Can you work these out from the model? Positions are in its coordinate system, mm. Face numbers are marked on the shaded views. A direction names the side the tool comes from. Give positions to 0.01 mm unless a question says otherwise; leave off trailing zeros. Order: outer loops, then holes, each group sorted by start corner. A loop starts at its lowest first (then second) coordinate and runs counter-clockwise, first axis right, second up. Notation, with made-up numbers: (67.5, -7.5) - (103.5, -7.5) arc R26 cw to (103.5, 15.5) - close; hole circle Ø10 at (12.5, -15). An arc over 180 degrees is marked (long way). Write each question's results on one line, items separated by ' | '. Start each with the question number.
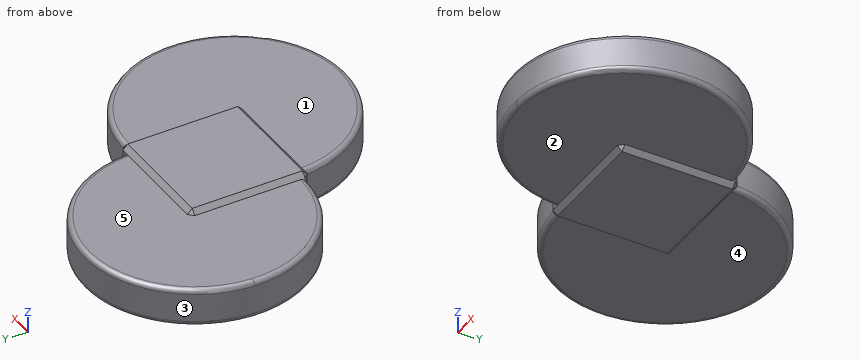
from build123d import *

# Parameters (mm, degrees)
F0_W          = 254
F0_H          = 254
F1_DEPTH      = 50.8
F1_DEPTH_BACK = 50.8
F2_SIZE       = 10.16
F1_FACE_W     = 233.68
F1_FACE_H     = 81.28
F1_FACE1_W    = 233.68
F1_FACE1_H    = 81.28
F5_T4_ANGLE   = 280.0079997231
F5_T9_ANGLE   = 280.0079997231
F5_T14_ANGLE  = 280.0079997231
F5_T19_ANGLE  = 280.0079997231
F5_T24_ANGLE  = 280.0079997231
F5_T29_ANGLE  = 280.0079997231
F5_T34_ANGLE  = 280.0079997231
F5_T39_ANGLE  = 280.0079997231
F5_T44_ANGLE  = 280.0079997231
F5_T49_ANGLE  = 280.0079997231
F5_T54_ANGLE  = 280.0079997231
F5_T59_ANGLE  = 280.0079997231


# Not quite as in the source:
# - a fillet or chamfer that OpenCascade refuses, or shapes differently, is made with other operations: its cross-section is extruded or revolved along the edge and cut away or added


with BuildPart() as f1:
    # F0 (on Top) → F1 (new body, two sides)
    with BuildSketch(Plane.XY) as f1_sk:
        Rectangle(F0_W, F0_H)
    extrude(amount=F1_DEPTH)
    extrude(f1_sk.sketch, amount=-F1_DEPTH_BACK)

    # F2
    f2_edges = [f1.edges().sort_by_distance(p)[0] for p in [
        (0, -127, 50.8),
        (127, -127, 0),
        (127, 0, 50.8),
        (-127, -127, 0),
        (0, -127, -50.8),
        (127, 0, -50.8),
        (127, 127, 0),
        (-127, 0, 50.8),
        (-127, 0, -50.8),
        (-127, 127, 0),
        (0, 127, 50.8),
        (0, 127, -50.8),
    ]]
    chamfer(f2_edges, length=F2_SIZE)

    # F1_face (on face) → F3 (revolve)
    with BuildSketch(Plane.YZ.offset(127)):
        Rectangle(F1_FACE_W, F1_FACE_H)
    revolve(axis=Axis((127, -116.84, 0), (0, 0, -1)))

    # F1_face1 (on face) → F4 (revolve)
    with BuildSketch(Plane(origin=(-127, 0, 0), x_dir=(0, -1, 0), z_dir=(-1, 0, 0))):
        Rectangle(F1_FACE1_W, F1_FACE1_H)
    revolve(axis=Axis((-127, 116.84, 0), (0, 0, 1)))

    # F5: fillet of radius 10.16 on 4 edges, made by hand


with BuildPart() as f5_tool2:
    # F5_s3 → F5_t4 (revolve)
    with BuildSketch(Plane(origin=(112.850510213, 12.3590473355, 0), x_dir=(0, 0, 1), z_dir=(-0.9940564274, -0.1088660602, 0))):
        with BuildLine():
            ThreePointArc((30.48, 103.70845737), (37.6642048969, 100.7326622668), (40.64, 93.54845737))
            Line((40.64, 93.54845737), (40.64, 103.70845737))
            Line((40.64, 103.70845737), (30.48, 103.70845737))
        make_face()
    revolve(axis=Axis((127, -116.84, 40.64), (0, 0, -1)), revolution_arc=F5_T4_ANGLE)

    split(bisect_by=Plane(origin=(83.82, 0, 83.82), x_dir=(0, 1, 0), z_dir=(0.7071067812, 0, 0.7071067812)), keep=Keep.TOP)


with BuildPart() as f1_1:
    add(f1.part)

    # F5_t1: cut F5_tool2
    add(f5_tool2.part, mode=Mode.SUBTRACT)


with BuildPart() as f5_tool7:
    # F5_s8 → F5_t9 (revolve)
    with BuildSketch(Plane(origin=(112.850510213, 12.3590473355, 0), x_dir=(0, 0, 1), z_dir=(-0.9940564274, -0.1088660602, 0))):
        with BuildLine():
            ThreePointArc((30.48, 103.70845737), (37.6642048969, 100.7326622668), (40.64, 93.54845737))
            Line((40.64, 93.54845737), (40.64, 103.70845737))
            Line((40.64, 103.70845737), (30.48, 103.70845737))
        make_face()
    revolve(axis=Axis((127, -116.84, 40.64), (0, 0, -1)), revolution_arc=F5_T9_ANGLE)

    split(bisect_by=Plane(origin=(121.92, 121.92, 0), x_dir=(0, 0, 1), z_dir=(0.7071067812, 0.7071067812, 0)), keep=Keep.TOP)


with BuildPart() as f1_2:
    add(f1_1.part)

    # F5_t6: cut F5_tool7
    add(f5_tool7.part, mode=Mode.SUBTRACT)


with BuildPart() as f5_tool12:
    # F5_s13 → F5_t14 (revolve)
    with BuildSketch(Plane(origin=(112.850510213, 12.3590473355, 0), x_dir=(0, 0, 1), z_dir=(-0.9940564274, -0.1088660602, 0))):
        with BuildLine():
            ThreePointArc((30.48, 103.70845737), (37.6642048969, 100.7326622668), (40.64, 93.54845737))
            Line((40.64, 93.54845737), (40.64, 103.70845737))
            Line((40.64, 103.70845737), (30.48, 103.70845737))
        make_face()
    revolve(axis=Axis((127, -116.84, 40.64), (0, 0, -1)), revolution_arc=F5_T14_ANGLE)

    split(bisect_by=Plane.XZ.offset(127), keep=Keep.TOP)


with BuildPart() as f1_3:
    add(f1_2.part)

    # F5_t11: cut F5_tool12
    add(f5_tool12.part, mode=Mode.SUBTRACT)


with BuildPart() as f5_tool17:
    # F5_s18 → F5_t19 (revolve)
    with BuildSketch(Plane(origin=(112.850510213, 12.3590473355, 0), x_dir=(0, 0, 1), z_dir=(-0.9940564274, -0.1088660602, 0))):
        with BuildLine():
            ThreePointArc((-30.48, 103.70845737), (-37.6642048969, 100.7326622668), (-40.64, 93.54845737))
            Line((-40.64, 93.54845737), (-40.64, 103.70845737))
            Line((-40.64, 103.70845737), (-30.48, 103.70845737))
        make_face()
    revolve(axis=Axis((127, -116.84, -40.64), (0, 0, -1)), revolution_arc=F5_T19_ANGLE)

    split(bisect_by=Plane(origin=(83.82, 0, -83.82), x_dir=(0, 1, 0), z_dir=(0.7071067812, 0, -0.7071067812)), keep=Keep.TOP)


with BuildPart() as f1_4:
    add(f1_3.part)

    # F5_t16: cut F5_tool17
    add(f5_tool17.part, mode=Mode.SUBTRACT)


with BuildPart() as f5_tool22:
    # F5_s23 → F5_t24 (revolve)
    with BuildSketch(Plane(origin=(112.850510213, 12.3590473355, 0), x_dir=(0, 0, 1), z_dir=(-0.9940564274, -0.1088660602, 0))):
        with BuildLine():
            ThreePointArc((-30.48, 103.70845737), (-37.6642048969, 100.7326622668), (-40.64, 93.54845737))
            Line((-40.64, 93.54845737), (-40.64, 103.70845737))
            Line((-40.64, 103.70845737), (-30.48, 103.70845737))
        make_face()
    revolve(axis=Axis((127, -116.84, -40.64), (0, 0, -1)), revolution_arc=F5_T24_ANGLE)

    split(bisect_by=Plane(origin=(121.92, 121.92, 0), x_dir=(0, 0, 1), z_dir=(0.7071067812, 0.7071067812, 0)), keep=Keep.TOP)


with BuildPart() as f1_5:
    add(f1_4.part)

    # F5_t21: cut F5_tool22
    add(f5_tool22.part, mode=Mode.SUBTRACT)


with BuildPart() as f5_tool27:
    # F5_s28 → F5_t29 (revolve)
    with BuildSketch(Plane(origin=(112.850510213, 12.3590473355, 0), x_dir=(0, 0, 1), z_dir=(-0.9940564274, -0.1088660602, 0))):
        with BuildLine():
            ThreePointArc((-30.48, 103.70845737), (-37.6642048969, 100.7326622668), (-40.64, 93.54845737))
            Line((-40.64, 93.54845737), (-40.64, 103.70845737))
            Line((-40.64, 103.70845737), (-30.48, 103.70845737))
        make_face()
    revolve(axis=Axis((127, -116.84, -40.64), (0, 0, -1)), revolution_arc=F5_T29_ANGLE)

    split(bisect_by=Plane.XZ.offset(127), keep=Keep.TOP)


with BuildPart() as f1_6:
    add(f1_5.part)

    # F5_t26: cut F5_tool27
    add(f5_tool27.part, mode=Mode.SUBTRACT)


with BuildPart() as f5_tool32:
    # F5_s33 → F5_t34 (revolve)
    with BuildSketch(Plane(origin=(7.0960267411, 108.0319683984, 0), x_dir=(0, 0, 1), z_dir=(-0.0655432689, -0.9978497281, 0))):
        with BuildLine():
            ThreePointArc((-30.48, -99.2950089912), (-37.6642048969, -96.319213888), (-40.64, -89.1350089912))
            Line((-40.64, -89.1350089912), (-40.64, -99.2950089912))
            Line((-40.64, -99.2950089912), (-30.48, -99.2950089912))
        make_face()
    revolve(axis=Axis((-127, 116.84, -40.64), (0, 0, 1)), revolution_arc=F5_T34_ANGLE)

    split(bisect_by=Plane.XZ.offset(-127), keep=Keep.BOTTOM)


with BuildPart() as f1_7:
    add(f1_6.part)

    # F5_t31: cut F5_tool32
    add(f5_tool32.part, mode=Mode.SUBTRACT)


with BuildPart() as f5_tool37:
    # F5_s38 → F5_t39 (revolve)
    with BuildSketch(Plane(origin=(7.0960267411, 108.0319683984, 0), x_dir=(0, 0, 1), z_dir=(-0.0655432689, -0.9978497281, 0))):
        with BuildLine():
            ThreePointArc((-30.48, -99.2950089912), (-37.6642048969, -96.319213888), (-40.64, -89.1350089912))
            Line((-40.64, -89.1350089912), (-40.64, -99.2950089912))
            Line((-40.64, -99.2950089912), (-30.48, -99.2950089912))
        make_face()
    revolve(axis=Axis((-127, 116.84, -40.64), (0, 0, 1)), revolution_arc=F5_T39_ANGLE)

    split(bisect_by=Plane(origin=(-83.82, 0, -83.82), x_dir=(0, 1, 0), z_dir=(-0.7071067812, 0, -0.7071067812)), keep=Keep.TOP)


with BuildPart() as f1_8:
    add(f1_7.part)

    # F5_t36: cut F5_tool37
    add(f5_tool37.part, mode=Mode.SUBTRACT)


with BuildPart() as f5_tool42:
    # F5_s43 → F5_t44 (revolve)
    with BuildSketch(Plane(origin=(7.0960267411, 108.0319683984, 0), x_dir=(0, 0, 1), z_dir=(-0.0655432689, -0.9978497281, 0))):
        with BuildLine():
            ThreePointArc((-30.48, -99.2950089912), (-37.6642048969, -96.319213888), (-40.64, -89.1350089912))
            Line((-40.64, -89.1350089912), (-40.64, -99.2950089912))
            Line((-40.64, -99.2950089912), (-30.48, -99.2950089912))
        make_face()
    revolve(axis=Axis((-127, 116.84, -40.64), (0, 0, 1)), revolution_arc=F5_T44_ANGLE)

    split(bisect_by=Plane(origin=(-121.92, -121.92, 0), x_dir=(0, 0, 1), z_dir=(-0.7071067812, -0.7071067812, 0)), keep=Keep.TOP)


with BuildPart() as f1_9:
    add(f1_8.part)

    # F5_t41: cut F5_tool42
    add(f5_tool42.part, mode=Mode.SUBTRACT)


with BuildPart() as f5_tool47:
    # F5_s48 → F5_t49 (revolve)
    with BuildSketch(Plane(origin=(7.0960267411, 108.0319683984, 0), x_dir=(0, 0, 1), z_dir=(-0.0655432689, -0.9978497281, 0))):
        with BuildLine():
            ThreePointArc((30.48, -99.2950089912), (37.6642048969, -96.319213888), (40.64, -89.1350089912))
            Line((40.64, -89.1350089912), (40.64, -99.2950089912))
            Line((40.64, -99.2950089912), (30.48, -99.2950089912))
        make_face()
    revolve(axis=Axis((-127, 116.84, 40.64), (0, 0, 1)), revolution_arc=F5_T49_ANGLE)

    split(bisect_by=Plane.XZ.offset(-127), keep=Keep.BOTTOM)


with BuildPart() as f1_10:
    add(f1_9.part)

    # F5_t46: cut F5_tool47
    add(f5_tool47.part, mode=Mode.SUBTRACT)


with BuildPart() as f5_tool52:
    # F5_s53 → F5_t54 (revolve)
    with BuildSketch(Plane(origin=(7.0960267411, 108.0319683984, 0), x_dir=(0, 0, 1), z_dir=(-0.0655432689, -0.9978497281, 0))):
        with BuildLine():
            ThreePointArc((30.48, -99.2950089912), (37.6642048969, -96.319213888), (40.64, -89.1350089912))
            Line((40.64, -89.1350089912), (40.64, -99.2950089912))
            Line((40.64, -99.2950089912), (30.48, -99.2950089912))
        make_face()
    revolve(axis=Axis((-127, 116.84, 40.64), (0, 0, 1)), revolution_arc=F5_T54_ANGLE)

    split(bisect_by=Plane(origin=(-83.82, 0, 83.82), x_dir=(0, 1, 0), z_dir=(-0.7071067812, 0, 0.7071067812)), keep=Keep.TOP)


with BuildPart() as f1_11:
    add(f1_10.part)

    # F5_t51: cut F5_tool52
    add(f5_tool52.part, mode=Mode.SUBTRACT)


with BuildPart() as f5_tool57:
    # F5_s58 → F5_t59 (revolve)
    with BuildSketch(Plane(origin=(7.0960267411, 108.0319683984, 0), x_dir=(0, 0, 1), z_dir=(-0.0655432689, -0.9978497281, 0))):
        with BuildLine():
            ThreePointArc((30.48, -99.2950089912), (37.6642048969, -96.319213888), (40.64, -89.1350089912))
            Line((40.64, -89.1350089912), (40.64, -99.2950089912))
            Line((40.64, -99.2950089912), (30.48, -99.2950089912))
        make_face()
    revolve(axis=Axis((-127, 116.84, 40.64), (0, 0, 1)), revolution_arc=F5_T59_ANGLE)

    split(bisect_by=Plane(origin=(-121.92, -121.92, 0), x_dir=(0, 0, 1), z_dir=(-0.7071067812, -0.7071067812, 0)), keep=Keep.TOP)


with BuildPart() as f1_12:
    add(f1_11.part)

    # F5_t56: cut F5_tool57
    add(f5_tool57.part, mode=Mode.SUBTRACT)


solid = f1_12.part
Q1. Which directions (+Z, -Z, +X, -X, +Y, -Y) give clear straight access to the entire face, cutting with the end or side of a thin tool? Please do the marked faces 1, 2, 3, 4 and 5.
Q2. If we section it at A-A (z = -21.5): Please give me the cut outline in (x, y), plus the area to 3 significant figures.
Q3. Will these pins go through, and if not, where does the flat tip stop? P1, Ø6, axis at x = 29.5, z = -14, coming from the -Y side; P2, Ø1.5, axis at x = 85, z = 6.5, coming from the +Y side; P3, Ø5, axis at x = -286, z = -2.5, coming from the +Y side.
Q4. If I drill on probe 1 along Z at (x, y) = (21, -170.5); probe 2 along X at (y, z) = (-277.5, 12); probe 3 along Y at (x, z) = (-139, -33), over which ranges is the centre line in solid material (lowest first)? Write a range as from..to.
Findings below:
1) face 1: +Z, +X, -Y | face 2: -Z, +X, -Y | face 3: +Z, -Z | face 4: -Z, -X, +Y | face 5: +Z, -X, +Y
2) outline: (-127, -116.84) - (-116.84, -127) - (-106.46, -127) arc R233.68 ccw (long way) to (127, 116.84) - (116.84, 127) - (106.46, 127) arc R233.68 ccw (long way) to start | area: 317,000 mm2
3) P1: stops at y = -330.56 | P2: stops at y = 216.74 | P3: stops at y = 290.37
4) probe 1: z = -40.64..40.64 | probe 2: x = -42.69..296.69 | probe 3: y = -116.21..349.89
